Geometry: final body of the model. Coordinates: model frame, mm. A direction names the side the tool comes from. Round coordinates to 2 decimals unless told otherwise and drop trailing zeros. Loops run counter-clockwise (first coordinate to the right, second up) from the corner with the lowest first, then second, coordinate; pieces in that order, holes last. Notation, with made-up numbers: (44.5, 22.25) -> (100.5, 22.25) arc R25 ccw to (100.5, 45.25) -> close; hole circle Ø2 at (84, -1.5). An arc over 180 degrees is marked (long way). Answer in a Markdown table with one row per item.
```python
from build123d import *

# Parameters (mm, degrees)
SKETCH_1_W          = 140
SKETCH_1_H          = 56
SKETCH_1_R          = 1.325
EXTRUDE_1_DEPTH     = 2
SKETCH_3_W          = 20.5
SKETCH_3_H          = 42
SKETCH_3_W_2        = 6
CUT_EXTRUDE_1_DEPTH = 10
FILLET_1_R          = 3
FILLET_2_R          = 2
FILLET_3_R          = 3
FILLET_4_R          = 5
CUT_EXTRUDE_2_DEPTH = 76.41883054
FILLET_5_R          = 2


with BuildPart() as part:
    # 草图1 → 凸台-拉伸1 (new body)
    with BuildSketch(Plane(origin=(0, 0, 0), x_dir=(1, 0, 0), z_dir=(0, 1, 0))):
        Rectangle(SKETCH_1_W, SKETCH_1_H)
        with Locations(Location((-65, 24, 0), (0, 0, 270))):
            Circle(SKETCH_1_R, mode=Mode.SUBTRACT)
        with Locations(Location((65, 24, 0), (0, 0, 270))):
            Circle(SKETCH_1_R, mode=Mode.SUBTRACT)
        with Locations(Location((65, -24, 0), (0, 0, 270))):
            Circle(SKETCH_1_R, mode=Mode.SUBTRACT)
        with Locations(Location((-65, -24, 0), (0, 0, 270))):
            Circle(SKETCH_1_R, mode=Mode.SUBTRACT)
    extrude(amount=EXTRUDE_1_DEPTH)

    # 草图3 → 切除-拉伸1 (cut)
    with BuildSketch(Plane(origin=(0, 2, 0), x_dir=(1, 0, 0), z_dir=(0, 1, 0))):
        with Locations((-49.75, 0)):
            Rectangle(SKETCH_3_W, SKETCH_3_H)
        with Locations((-65, 0)):
            Rectangle(SKETCH_3_W_2, SKETCH_3_H)
        Polygon((-36.5, -22.50398901), (-2.275183381, 0), (-36.5, 22.50398901), align=None)
        Polygon((34.224816619, 24), (-34.224816619, 24), (0, 1.49601099), align=None)
        Polygon((36.5, 22.50398901), (2.275183381, 0), (36.5, -22.50398901), align=None)
        Polygon((34.224816619, -24), (0, -1.49601099), (-34.224816619, -24), align=None)
        with Locations((49.75, 0)):
            Rectangle(SKETCH_3_W, SKETCH_3_H)
        with Locations((65, 0)):
            Rectangle(SKETCH_3_W_2, SKETCH_3_H)
    extrude(amount=-CUT_EXTRUDE_1_DEPTH, mode=Mode.SUBTRACT)

    # 圆角1
    fillet_1_edges = [part.edges().sort_by_distance(p)[0] for p in [
        (68, 1, -21),
        (68, 1, 21),
        (62, 1, 21),
        (62, 1, -21),
        (-60, 1, 21),
        (-60, 1, -21),
        (-39.5, 1, -21),
        (-39.5, 1, 21),
        (70, 1, 28),
        (-70, 1, 28),
        (-70, 1, -28),
        (70, 1, -28),
        (-62, 1, -21),
        (-62, 1, 21),
        (-68, 1, 21),
        (-68, 1, -21),
        (60, 1, -21),
        (60, 1, 21),
        (39.5, 1, 21),
        (39.5, 1, -21),
    ]]
    fillet(fillet_1_edges, radius=FILLET_1_R - 0.0001)  # a hair under: the kernel refuses the full size

    # 圆角2
    fillet_2_edges = [part.edges().sort_by_distance(p)[0] for p in [
        (-34.224816619, 1, -24),
        (34.224816619, 1, -24),
        (2.275183381, 1, 0),
        (-2.275183381, 1, 0),
        (-34.224816619, 1, 24),
        (34.224816619, 1, 24),
    ]]
    fillet(fillet_2_edges, radius=FILLET_2_R)

    # 圆角3
    fillet_3_edges = [part.edges().sort_by_distance(p)[0] for p in [
        (36.5, 1, -22.50398901),
        (36.5, 1, 22.50398901),
        (-36.5, 1, -22.50398901),
        (-36.5, 1, 22.50398901),
    ]]
    fillet(fillet_3_edges, radius=FILLET_3_R)

    # 圆角4
    fillet_4_edges = [part.edges().sort_by_distance(p)[0] for p in [
        (0, 1, -1.49601099),
        (0, 1, 1.49601099),
    ]]
    fillet(fillet_4_edges, radius=FILLET_4_R)

    # 草图4 → 切除-拉伸2 (cut, through all)
    with BuildSketch(Plane(origin=(0, 2, 0), x_dir=(1, 0, 0), z_dir=(0, 1, 0))):
        Polygon((-41.020833333, 28), (-39.5, 27), (39.5, 27), (41.020833333, 28), align=None)
        Polygon((41.020833333, -28), (39.5, -27), (-39.5, -27), (-41.020833333, -28), align=None)
    extrude(amount=-CUT_EXTRUDE_2_DEPTH, mode=Mode.SUBTRACT)

    # 圆角5
    fillet_5_edges = [part.edges().sort_by_distance(p)[0] for p in [
        (-41.020833333, 1, -28),
        (41.020833333, 1, -28),
        (39.5, 1, -27),
        (-39.5, 1, -27),
        (41.020833333, 1, 28),
        (-41.020833333, 1, 28),
        (-39.5, 1, 27),
        (39.5, 1, 27),
    ]]
    fillet(fillet_5_edges, radius=FILLET_5_R)


solid = part.part
```
Item 1: Section query B-B, the plane z = 0. Output: boundary loops of the cut face in (x, y), and give its area (3 significant figures).
Ans:
| item | result |
|---|---|
| outline | (-70, 0) -> (-68, 0) -> (-68, 2) -> (-70, 2) -> close; (-62, 0) -> (-60, 0) -> (-60, 2) -> (-62, 2) -> close; (-39.5, 0) -> (-36.5, 0) -> (-36.5, 2) -> (-39.5, 2) -> close; (-3.92, 0) -> (3.92, 0) -> (3.92, 2) -> (-3.92, 2) -> close; (36.5, 0) -> (39.5, 0) -> (39.5, 2) -> (36.5, 2) -> close; (60, 0) -> (62, 0) -> (62, 2) -> (60, 2) -> close; (68, 0) -> (70, 0) -> (70, 2) -> (68, 2) -> close |
| area | 43.7 mm2 |
Item 2: Section query A-A, the plane x = -54.5. Output: boundary loops of the cut face in (y, z), and give its area (3 significant figures).
Ans:
| item | result |
|---|---|
| outline | (0, -28) -> (2, -28) -> (2, -21) -> (0, -21) -> close; (0, 21) -> (2, 21) -> (2, 28) -> (0, 28) -> close |
| area | 28.0 mm2 |
Item 3: First-contact query: P1, Ø1, axis at x = 29.5, y = 1, coming from the +Z side; P2, Ø0.6, axis at x = 1.5, y = 1, coming from the -Z side. Flat tips, straight axial feed; report the tip coordinate or a pass-through.
Ans:
| item | result |
|---|---|
| P1 | z = 27 |
| P2 | z = -27 |
Item 4: Set-up query: faces 4 (the cylindrical face through (67.14, 0.99, -20.1)), 5 (the cylindrical face through (-69.14, 1.01, 27.1)). Return all of +Z, -Z, +X, -X, +Y, -Y with unobstructed straight access to the full face (end or side cutting, diameter ignored); none if empty.
Ans:
| item | result |
|---|---|
| face 4 | +Y, -Y |
| face 5 | +Z, -X, +Y, -Y |
Item 5: Section query C-C, the plane z = -11.5. State how many separate pieces and enclosed holes the cut face has, and give its area (3 significant figures).
Ans:
| item | result |
|---|---|
| separate pieces | 8 |
| enclosed holes | 0 |
| area | 46.2 mm2 |
Item 6: Mould query, pull axis X, two halves, no side actions, for faces 1 (the cylindrical face through (-66.293, 0.986, 23.713)), 2 (the cylindrical face through (-69.14, 1.01, -27.1)), 3 (the cylindrical face through (69.1, 1.01, 27.14)). Classes: released by +X, released by -X, zero draft, split by the parting line, or undercut.
Ans:
| item | result |
|---|---|
| face 1 | undercut |
| face 2 | released by -X |
| face 3 | released by +X |
Item 7: Ray query, L1, parallel to Z at x = -65, y = 0.85 (3 decimals); L2, parallel to Z at x = -55, y = 0.55; L3, parallel to Z at x = 17, y = 1.1. Return the intervals inside material, ascending.
Ans:
| item | result |
|---|---|
| L1 | -28 to -25.325, -22.675 to -21, 21 to 22.675, 25.325 to 28 |
| L2 | -28 to -21, 21 to 28 |
| L3 | -27 to -24, -12.67 to -9.68, 9.68 to 12.67, 24 to 27 |
Item 8: Section query D-D, the plane x = 9. Output: boundary loops of the cut face in (y, z).
Ans:
| item | result |
|---|---|
| outline | (0, -27) -> (2, -27) -> (2, -24) -> (0, -24) -> close; (0, -7.41) -> (2, -7.41) -> (2, -4.42) -> (0, -4.42) -> close; (0, 4.42) -> (2, 4.42) -> (2, 7.41) -> (0, 7.41) -> close; (0, 24) -> (2, 24) -> (2, 27) -> (0, 27) -> close |
